```python
from build123d import *

# Parameters (mm, degrees)
SKETCH1_R           = 101.6
BOSS_EXTRUDE2_DEPTH = 76.2
SKETCH2_R           = 21.59
CUT_EXTRUDE1_DEPTH  = 76.2


with BuildPart() as part:
    # Sketch1 → Boss-Extrude2 (new body)
    with BuildSketch(Plane(origin=(0, 0, 0), x_dir=(1, 0, 0), z_dir=(0, 1, 0))):
        Circle(SKETCH1_R)
        with BuildLine():
            Line((36.477972806, 0), (64.570477, 0))
            ThreePointArc((64.570477, 0), (68.300787401, 1.631640344), (69.634828137, 5.478431373))
            ThreePointArc((69.634828137, 5.478431373), (65.706637707, 23.699372591), (57.099502026, 40.232690295))
            ThreePointArc((57.099502026, 40.232690295), (53.382107886, 42.367992154), (49.354708521, 40.898778904))
            Line((49.354708521, 40.898778904), (29.068878602, 20.612948985))
            ThreePointArc((29.068878602, 20.612948985), (27.639931466, 17.792507776), (28.156018147, 14.673143566))
            ThreePointArc((28.156018147, 14.673143566), (30.242464115, 9.667257328), (31.446528281, 4.379310345))
            ThreePointArc((31.446528281, 4.379310345), (33.142789411, 1.24816601), (36.477972806, 0))
        make_face(mode=Mode.SUBTRACT)
        with BuildLine():
            Line((32.385776769, -14.867912836), (60.096735775, -22.293041923))
            ThreePointArc((60.096735775, -22.293041923), (63.382811455, -25.04626546), (63.392282871, -29.33327415))
            ThreePointArc((63.392282871, -29.33327415), (53.377577571, -45.053931156), (39.56187481, -57.566314469))
            ThreePointArc((39.56187481, -57.566314469), (35.563435689, -58.334396815), (32.2852385, -55.919673416))
            Line((32.2852385, -55.919673416), (18.238986403, -31.590851128))
            ThreePointArc((18.238986403, -31.590851128), (17.652338179, -28.078414577), (19.51585815, -25.043837179))
            ThreePointArc((19.51585815, -25.043837179), (23.493322488, -21.357113533), (26.785324155, -17.047255202))
            ThreePointArc((26.785324155, -17.047255202), (29.228729464, -15.04062892), (32.385776769, -14.867912836))
        make_face(mode=Mode.SUBTRACT)
        with BuildLine():
            Line((3.316898167, -35.480861821), (10.742027254, -63.191820828))
            ThreePointArc((10.742027254, -63.191820828), (10.00070357, -67.414257614), (6.292780846, -69.565964445))
            ThreePointArc((6.292780846, -69.565964445), (-12.329060136, -68.753303747), (-30.072953327, -63.044745841))
            ThreePointArc((-30.072953327, -63.044745841), (-32.737351712, -59.96603716), (-32.2852385, -55.919673416))
            Line((-32.2852385, -55.919673416), (-18.238986403, -31.590851128))
            ThreePointArc((-18.238986403, -31.590851128), (-15.490451232, -29.326580587), (-11.930670131, -29.423147524))
            ThreePointArc((-11.930670131, -29.423147524), (-6.749141627, -31.024370861), (-1.370693992, -31.720398768))
            ThreePointArc((-1.370693992, -31.720398768), (1.588797998, -32.833136696), (3.316898167, -35.480861821))
        make_face(mode=Mode.SUBTRACT)
        with BuildLine():
            Line((-29.068878602, -20.612948985), (-49.354708521, -40.898778904))
            ThreePointArc((-49.354708521, -40.898778904), (-53.382107886, -42.367992154), (-57.099502026, -40.232690295))
            ThreePointArc((-57.099502026, -40.232690295), (-65.706637707, -23.699372591), (-69.634828137, -5.478431373))
            ThreePointArc((-69.634828137, -5.478431373), (-68.300787401, -1.631640344), (-64.570477, 0))
            Line((-64.570477, 0), (-36.477972806, 0))
            ThreePointArc((-36.477972806, 0), (-33.142789411, -1.24816601), (-31.446528281, -4.379310345))
            ThreePointArc((-31.446528281, -4.379310345), (-30.242464115, -9.667257328), (-28.156018147, -14.673143566))
            ThreePointArc((-28.156018147, -14.673143566), (-27.639931466, -17.792507776), (-29.068878602, -20.612948985))
        make_face(mode=Mode.SUBTRACT)
        with BuildLine():
            Line((-32.385776769, 14.867912836), (-60.096735775, 22.293041923))
            ThreePointArc((-60.096735775, 22.293041923), (-63.382811455, 25.04626546), (-63.392282871, 29.33327415))
            ThreePointArc((-63.392282871, 29.33327415), (-53.377577571, 45.053931156), (-39.56187481, 57.566314469))
            ThreePointArc((-39.56187481, 57.566314469), (-35.563435689, 58.334396815), (-32.2852385, 55.919673416))
            Line((-32.2852385, 55.919673416), (-18.238986403, 31.590851128))
            ThreePointArc((-18.238986403, 31.590851128), (-17.652338179, 28.078414577), (-19.51585815, 25.043837179))
            ThreePointArc((-19.51585815, 25.043837179), (-23.493322488, 21.357113533), (-26.785324155, 17.047255202))
            ThreePointArc((-26.785324155, 17.047255202), (-29.228729464, 15.04062892), (-32.385776769, 14.867912836))
        make_face(mode=Mode.SUBTRACT)
        with BuildLine():
            Line((-3.316898167, 35.480861821), (-10.742027254, 63.191820828))
            ThreePointArc((-10.742027254, 63.191820828), (-10.00070357, 67.414257614), (-6.292780846, 69.565964445))
            ThreePointArc((-6.292780846, 69.565964445), (12.329060136, 68.753303747), (30.072953327, 63.044745841))
            ThreePointArc((30.072953327, 63.044745841), (32.737351712, 59.96603716), (32.2852385, 55.919673416))
            Line((32.2852385, 55.919673416), (18.238986403, 31.590851128))
            ThreePointArc((18.238986403, 31.590851128), (15.490451232, 29.326580587), (11.930670131, 29.423147524))
            ThreePointArc((11.930670131, 29.423147524), (6.749141627, 31.024370861), (1.370693992, 31.720398768))
            ThreePointArc((1.370693992, 31.720398768), (-1.588797998, 32.833136696), (-3.316898167, 35.480861821))
        make_face(mode=Mode.SUBTRACT)
    extrude(amount=BOSS_EXTRUDE2_DEPTH)

    # Sketch2 → Cut-Extrude1 (cut)
    with BuildSketch(Plane(origin=(0, 76.2, 0), x_dir=(1, 0, 0), z_dir=(0, 1, 0))):
        Circle(SKETCH2_R)
    extrude(amount=-CUT_EXTRUDE1_DEPTH, mode=Mode.SUBTRACT)


solid = part.part
```
Check sheet for the modelled part. Datum: model origin and axes. Units: mm. Round coordinates to 2 decimals unless told otherwise and drop trailing zeros. Order: outer loops, then holes, each group sorted by start corner. A loop starts at its lowest first (then second) coordinate and runs counter-clockwise, first axis right, second up.
1) Go/stop test with flat-tipped pins: pin 1 Ø1 at (y, z) = (20, 11.5) entering from +X; pin 2 Ø10 at (y, z) = (36, 56) entering from -X; pin 3 Ø8 at (y, z) = (39.5, -69.5) entering from +X. Record where each tip stops, or that it passes through.
2) Scan lines: line 1 (Z direction, x = 0, y = 54.5); line 2 (X direction, y = 16, z = 5); line 3 (X direction, y = 10.5, z = -2). Record each from-to range of solid material in increasing order.
3) Mould release check, pull along X, two halves, no side actions. Record for faces 1 (the cylindrical face through (-15.913, 38.633, -14.592)), 2 (the flat face through (-24, 0, -1)), 3 (the cylindrical face through (-22.025, 37.567, 99.184)), 4 (the cylindrical face through (63.356, 37.567, 24.99)): +X half, -X half, draft (parallel to the pull), parting line (faces both ways), or undercut.
4) Section check A-A (z = -12). Record the boundary of the cut face in (x, y).
5) Section check B-B (y = 63). Give the number of separate pieces and of enclosed holes in the cut face, and give its area (3 significant figures).
6) Section check D-D (x = -74.5). Record the boundary of the cut face in (y, z).
7) Section check C-C (z = -51). Record the boundary of the cut face in (x, y).
Result:
1. pin 1: stops at x = 101
1. pin 2: stops at x = -87.87
1. pin 3: stops at x = 77.67
2. line 1: z = -101.6 to -69.85, -31.97 to -21.59, 21.59 to 31.97, 69.85 to 101.6
2. line 2: x = -101.48 to -69.65, -31.35 to -21, 21 to 101.48
2. line 3: x = -101.58 to -21.5, 21.5 to 32.44, 68.61 to 101.58
3. face 1: undercut
3. face 2: draft
3. face 3: parting line
3. face 4: undercut
4. outline: (-100.89, 0) - (-17.95, 0) - (-17.95, 76.2) - (-100.89, 76.2) - close; (17.95, 0) - (29.39, 0) - (29.39, 76.2) - (17.95, 76.2) - close; (68.81, 0) - (100.89, 0) - (100.89, 76.2) - (68.81, 76.2) - close
5. separate pieces: 1
5. enclosed holes: 7
5. area: 23,300 mm2
6. outline: (0, -69.08) - (76.2, -69.08) - (76.2, 69.08) - (0, 69.08) - close
7. outline: (-87.87, 0) - (-47.73, 0) - (-47.73, 76.2) - (-87.87, 76.2) - close; (-29.44, 0) - (-7.48, 0) - (-7.48, 76.2) - (-29.44, 76.2) - close; (29.44, 0) - (87.87, 0) - (87.87, 76.2) - (29.44, 76.2) - close
